```python
from build123d import *
from build123d.topology import SkipClean

# Parameters (mm, degrees)
BOSS_EXTRUDE1_DEPTH = 2
SKETCH2_R           = 4
CUT_EXTRUDE1_DEPTH  = 2
SKETCH3_W           = 10
SKETCH3_H           = 5
CUT_EXTRUDE2_DEPTH  = 10
SKETCH7_R           = 1.5
CUT_EXTRUDE3_DEPTH  = 10
SKETCH8_R           = 10.5
CUT_EXTRUDE4_DEPTH  = 101.478560353
BOSS_EXTRUDE2_DEPTH = 75
BOSS_EXTRUDE3_DEPTH = 2
BOSS_EXTRUDE4_DEPTH = 2


with BuildPart() as part:
    # Sketch1 → Boss-Extrude1 (new body)
    with BuildSketch(Plane(origin=(0, 0, 0), x_dir=(1, 0, 0), z_dir=(0, 1, 0))):
        with BuildLine():
            Line((-37.5, -63.919410907), (37.5, -63.919410907))
            Line((37.5, -63.919410907), (37.5, -13.919410907))
            ThreePointArc((37.5, -13.919410907), (0, 40), (-37.5, -13.919410907))
            Line((-37.5, -13.919410907), (-37.5, -63.919410907))
        make_face()
    extrude(amount=BOSS_EXTRUDE1_DEPTH)

    # Sketch2 → Cut-Extrude1 (cut)
    with BuildSketch(Plane(origin=(0, 2, 0), x_dir=(1, 0, 0), z_dir=(0, 1, 0))):
        with Locations(Location((0, 0, 0), (0, 0, 270))):
            Circle(SKETCH2_R)
    extrude(amount=-CUT_EXTRUDE1_DEPTH, mode=Mode.SUBTRACT)

    # Sketch3 → Cut-Extrude2 (cut)
    with BuildSketch(Plane(origin=(0, 2, 0), x_dir=(1, 0, 0), z_dir=(0, 1, 0))):
        with Locations((0, -22.5)):
            Rectangle(SKETCH3_W, SKETCH3_H)
    extrude(amount=-CUT_EXTRUDE2_DEPTH, mode=Mode.SUBTRACT)

    # Sketch7 → Cut-Extrude3 (cut)
    with BuildSketch(Plane(origin=(0, 2, 0), x_dir=(1, 0, 0), z_dir=(0, 1, 0))):
        with Locations(Location((0, 37, 0), (0, 0, 270))):
            Circle(SKETCH7_R)
        with Locations(Location((-34.5, -60.919410907, 0), (0, 0, 270))):
            Circle(SKETCH7_R)
        with Locations(Location((34.5, -60.919410907, 0), (0, 0, 270))):
            Circle(SKETCH7_R)
    extrude(amount=-CUT_EXTRUDE3_DEPTH, mode=Mode.SUBTRACT)

    # Sketch8 → Cut-Extrude4 (cut, through all)
    with BuildSketch(Plane.ZY.offset(37.5)):
        with Locations((45.278815685, 0.949918898)):
            Circle(SKETCH8_R)
    extrude(amount=-CUT_EXTRUDE4_DEPTH, mode=Mode.SUBTRACT)


with BuildPart() as cut_extrude4_piece_1:
    # of the separate pieces the step leaves, piece 1, a body of its own (cut_extrude4_pieces)
    add(part.part.solids().sort_by_distance((-37.5, 0, 13.919410907))[0])



with BuildPart() as cut_extrude4_piece_2:
    # of the separate pieces the step leaves, piece 2, a body of its own (cut_extrude4_pieces)
    add(part.part.solids().sort_by_distance((-37.5, 0, 55.73575855))[0])


with BuildPart() as cut_extrude4_piece_1_1:
    with SkipClean():  # the faces are left unmerged after this step: merging them gives an invalid solid
        add(cut_extrude4_piece_1.part)

        add(cut_extrude4_piece_2.part)  # Boss-Extrude2 merges Cut-Extrude4 piece 2
        # Sketch9 → Boss-Extrude2 (add)
        with BuildSketch(Plane.ZY.offset(37.5)):
            with BuildLine():
                Line((32.814961783, 0), (34.821872819, 0))
                ThreePointArc((34.821872819, 0), (45.278815685, 11.449918898), (55.73575855, 0))
                Line((55.73575855, 0), (57.742669586, 0))
                ThreePointArc((57.742669586, 0), (45.278815685, 13.449918898), (32.814961783, 0))
            make_face()
        extrude(amount=-BOSS_EXTRUDE2_DEPTH)

    # Sketch10 → Boss-Extrude3 (add)
    with BuildSketch(Plane.ZY.offset(37.5)):
        with BuildLine():
            Line((32.814961783, 0), (57.742669586, 0))
            ThreePointArc((57.742669586, 0), (45.278815685, 13.449918898), (32.814961783, 0))
        make_face()
    extrude(amount=-BOSS_EXTRUDE3_DEPTH)

    # Sketch11 → Boss-Extrude4 (add)
    with SkipClean():  # the faces are left unmerged after this step: merging them gives an invalid solid
        with BuildSketch(Plane(origin=(37.5, 0, 0), x_dir=(0, 0, -1), z_dir=(1, 0, 0))):
            with BuildLine():
                Line((-57.742669586, 0), (-32.814961783, 0))
                ThreePointArc((-32.814961783, 0), (-45.278815685, 13.449918898), (-57.742669586, 0))
            make_face()
        extrude(amount=-BOSS_EXTRUDE4_DEPTH)


solid = cut_extrude4_piece_1_1.part
```
Geometry: final body of the model. Coordinates: model frame, mm. A direction names the side the tool comes from. Coordinates: 2 decimals unless noted, no trailing zeros. Order: outer loops, then holes, each group sorted by start corner. A loop starts at its lowest first (then second) coordinate and runs counter-clockwise, first axis right, second up. Notation, with made-up numbers: (21.25, 46) -> (77.25, 46) arc R11 cw to (77.25, 59) -> close; hole circle Ø11 at (19, -18). An arc over 180 degrees is marked (long way). Answer in a Markdown table with one row per item.
Item 1: Section B-B on z = -37. Output: boundary loops of the cut face in (x, y), plus the area to 3 significant figures.
Return value:
| item | result |
|---|---|
| outline | (-15.2, 0) -> (-1.5, 0) -> (-1.5, 2) -> (-15.2, 2) -> close; (1.5, 0) -> (15.2, 0) -> (15.2, 2) -> (1.5, 2) -> close |
| area | 54.8 mm² |
Item 2: Section D-D on x = 0. Output: boundary loops of the cut face in (y, z), plus the area to 3 significant figures.
Return value:
| item | result |
|---|---|
| outline | (0, -40) -> (2, -40) -> (2, -38.5) -> (0, -38.5) -> close; (0, -35.5) -> (2, -35.5) -> (2, -4) -> (0, -4) -> close; (0, 4) -> (2, 4) -> (2, 20) -> (0, 20) -> close; (0, 25) -> (2, 25) -> (2, 32.82) arc R12.5 ccw to (2, 57.73) -> (2, 63.92) -> (0, 63.92) -> (0, 55.74) arc R10.5 cw (long way) to (0, 34.82) -> close |
| area | 202 mm² |
Item 3: Draft query along Z for faces 5 (the flat face through (-1, 0, 11)), 6 (the cylindrical face through (1.079, 0.986, -39.985)), 7 (the flat face through (0, 1, 20)). Return one class per face: released by +Z, released by -Z, zero draft, split by the parting line, or undercut.
Return value:
| item | result |
|---|---|
| face 5 | zero draft |
| face 6 | split by the parting line |
| face 7 | undercut |
Item 4: Access query for faces 1 (the flat face through (-37.5, 5, 44)), 2 (the flat face through (37.5, 5, 45)), 3 (the flat face through (-5, 1, 23)), 4 (the flat face through (-35.5, 5, 45)). Directions: +Z, -Z, +X, -X, +Y, -Y. A direction counts if a zero-diameter tool reaches every point of the face in a straight line with its end or side. Return the directions, or none.
Return value:
| item | result |
|---|---|
| face 1 | +Z, -X, +Y, -Y |
| face 2 | +Z, +X, +Y, -Y |
| face 3 | +Y, -Y |
| face 4 | -Y |
Item 5: Ray query, L1, parallel to X at y = 3, z = 47.5; L2, parallel to X at y = 1.3, z = 0; L3, parallel to Y at x = 12, z = 9.5. Return the intervals inside material, ascending.
Return value:
| item | result |
|---|---|
| L1 | x = -37.5 to -35.5, 35.5 to 37.5 |
| L2 | x = -40 to -4, 4 to 40 |
| L3 | y = 0 to 2 |
Item 6: Contact query for flat-ended pins moving along their axis: P1, Ø7, axis at x = 0, z = 0, coming from the -Y side; P2, Ø3, axis at x = 19.5, y = 9, coming from the +Z side; P3, Ø1, axis at x = -24, z = 28.5, coming from the +Y side; P4, Ø1, axis at y = 1, z = 21.5, coming from the +X side. Output: stop coordinate, or through.
Return value:
| item | result |
|---|---|
| P1 | passes through |
| P2 | stops at z = 55.93 |
| P3 | stops at y = 2 |
| P4 | stops at x = 37.5 |
Item 7: Section A-A on y = 6. Output: boundary loops of the cut face in (x, z), plus the area to 3 significant figures.
Return value:
| item | result |
|---|---|
| outline | (-37.5, 33.84) -> (37.5, 33.84) -> (37.5, 56.71) -> (-37.5, 56.71) -> close; hole (-35.5, 36.07) -> (35.5, 36.07) -> (35.5, 54.48) -> (-35.5, 54.48) -> close |
| area | 408 mm² |
Item 8: Section C-C on x = 20.5. Output: boundary loops of the cut face in (y, z).
Return value:
| item | result |
|---|---|
| outline | (0, -34.35) -> (2, -34.35) -> (2, 32.82) arc R12.5 ccw to (2, 57.73) -> (2, 63.92) -> (0, 63.92) -> (0, 55.74) arc R10.5 cw (long way) to (0, 34.82) -> close |
